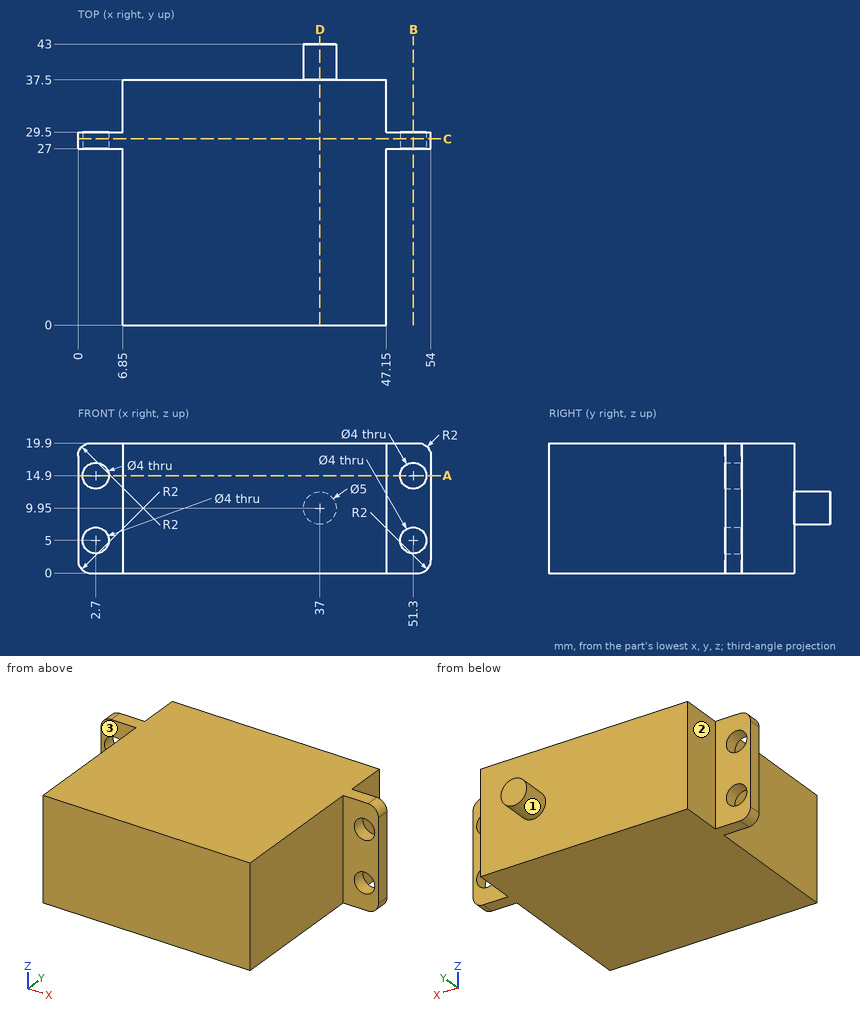
Job drawing, mm, ordinate dimensions from the low corner. One solid piece. A direction names the side the tool comes from. Coordinates: 2 decimals unless noted, no trailing zeros. Write each loop counter-clockwise with the first axis right and the second up, starting at its lowest first coordinate (ties: lowest second). Pieces come first, ordered by that corner, then holes.
Item 1: Pin check, flat tips, straight feed: pin 1 (4 mm diameter, centred on x = 47.5, z = 18, fed in from -Y); pin 2 (3.5 mm diameter, centred on x = 2.7, z = 5, fed in from +Y); pin 3 (2 mm diameter, centred on x = 2.5, z = 11, fed in from -Y); pin 4 (2.5 mm diameter, centred on y = 35, z = 12, fed in from +X). Stop position of each tip, or through.
Item 2: Which spindle directions (+Z, -Z, +X, -X, +Y, -Y) get a long thin tool onto all of the face, cutting with end or side? Do the marked faces 1, 2 and 3. Say none if no direction does.
Item 3: Slice it at A-A (z = 14.9). Write the cut outline in (x, y).
Item 4: Probe line 1 (X direction, y = 27.8, z = 5); line 2 (Z direction, x = 51, y = 28); line 3 (X direction, y = 12, z = 14.75). List the from-to ranges inside material, lowest first.
Item 5: Slice it at D-D (x = 37). Write the cut outline in (y, z), and give its area (3 significant figures).
Item 6: Slice it at B-B (x = 51.3). Write the cut outline in (y, z).
Item 7: Slice it at C-C (y = 28.5). Write the cut outline in (x, z), and give its area (3 significant figures).
Results found:
1. pin 1: stops at y = 0
1. pin 2: passes through
1. pin 3: stops at y = 27
1. pin 4: stops at x = 47.15
2. face 1: +Y
2. face 2: +Z, -Z, -X, +Y
2. face 3: +Z, -Z, -X, -Y
3. outline: (0, 27) - (0.7, 27) - (0.7, 29.5) - (0, 29.5) - close; (4.7, 27) - (6.85, 27) - (6.85, 0) - (47.15, 0) - (47.15, 27) - (49.3, 27) - (49.3, 29.5) - (47.15, 29.5) - (47.15, 37.5) - (6.85, 37.5) - (6.85, 29.5) - (4.7, 29.5) - close; (53.3, 27) - (54, 27) - (54, 29.5) - (53.3, 29.5) - close
4. line 1: x = 0 to 0.7, 4.7 to 49.3, 53.3 to 54
4. line 2: z = 0 to 3.02, 6.98 to 12.92, 16.88 to 19.9
4. line 3: x = 6.85 to 47.15
5. outline: (0, 0) - (37.5, 0) - (37.5, 7.45) - (43, 7.45) - (43, 12.45) - (37.5, 12.45) - (37.5, 19.9) - (0, 19.9) - close
5. area: 774 mm2
6. outline: (27, 0) - (29.5, 0) - (29.5, 3) - (27, 3) - close; (27, 7) - (29.5, 7) - (29.5, 12.9) - (27, 12.9) - close; (27, 16.9) - (29.5, 16.9) - (29.5, 19.9) - (27, 19.9) - close
7. outline: (0, 2) arc R2 ccw to (2, 0) - (52, 0) arc R2 ccw to (54, 2) - (54, 17.9) arc R2 ccw to (52, 19.9) - (2, 19.9) arc R2 ccw to (0, 17.9) - close; hole circle Ø4 at (2.7, 5); hole circle Ø4 at (2.7, 14.9); hole circle Ø4 at (51.3, 5); hole circle Ø4 at (51.3, 14.9)
7. area: 1,020 mm2
